from build123d import *

# Parameters (mm, degrees)
F0_W        = 105
F0_H        = 60
F1_DEPTH    = 20
F2_R        = 2.5
F3_R        = 2.5
F4_R        = 2.5
F5_T1_DEPTH = 23.75
F5_S5_W     = 2.5
F5_S5_H     = 2.5
F5_T6_DEPTH = 2.5
F6_R        = 2.5


# Not quite as in the source:
# - a fillet or chamfer that OpenCascade refuses, or shapes differently, is made with other operations: its cross-section is extruded or revolved along the edge and cut away or added


with BuildPart() as f1:
    # F0 (on Top) → F1 (new body)
    with BuildSketch(Plane.XY):
        Rectangle(F0_W, F0_H)
        with BuildLine():
            ThreePointArc((-17.4192723763, 1.0974504119), (-17.4394815095, 0.547242643), (-17.5, 0))
            ThreePointArc((-17.5, 0), (-32.3990632431, 1.6476581808), (-17.4192723763, 1.0974504119))
        make_face(mode=Mode.SUBTRACT)
        with BuildLine():
            ThreePointArc((-7.5, 0), (0, 7.5), (7.5, 0))
            ThreePointArc((7.5, 0), (0, -7.5), (-7.5, 0))
        make_face(mode=Mode.SUBTRACT)
        with BuildLine():
            ThreePointArc((32.4798090562, 0.5499604379), (25.2549745325, -6.9449901264), (17.5, 0))
            ThreePointArc((17.5, 0), (24.7046435799, 8.0449110021), (32.4798090562, 0.5499604379))
        make_face(mode=Mode.SUBTRACT)
    extrude(amount=F1_DEPTH)

    # F2
    f2_edges = [f1.edges().sort_by_distance(p)[0] for p in [
        (0, -30, 20),
    ]]
    fillet(f2_edges, radius=F2_R)

    # F3
    f3_edges = [f1.edges().sort_by_distance(p)[0] for p in [
        (52.5, 1.25, 20),
        (0, 30, 20),
    ]]
    fillet(f3_edges, radius=F3_R)

    # F4
    f4_edges = [f1.edges().sort_by_distance(p)[0] for p in [
        (-52.5, 0, 20),
    ]]
    fillet(f4_edges, radius=F4_R)

    # F5: fillet of radius 2.5 on 1 edges, made by hand

    # F5_s2 → F5_t1 (cut)
    with BuildSketch(Plane.XY.offset(-6.25)):
        with BuildLine():
            ThreePointArc((50, 30), (51.767766953, 29.267766953), (52.5, 27.5))
            Line((52.5, 27.5), (52.5, 30))
            Line((52.5, 30), (50, 30))
        make_face()
    extrude(amount=F5_T1_DEPTH, mode=Mode.SUBTRACT)


with BuildPart() as f5_tool4:
    # F5_s5 → F5_t6 (new body)
    with BuildSketch(Plane.XZ.offset(-27.5)):
        with Locations((51.25, 18.75)):
            Rectangle(F5_S5_W, F5_S5_H)
    extrude(amount=-F5_T6_DEPTH)

    # F5_s7 → F5_t8 (revolve, cut)
    with BuildSketch(Plane(origin=(50, 27.5, 17.5), x_dir=(-0.7071067812, 0, -0.7071067812), z_dir=(0.7071067812, 0, -0.7071067812))):
        with BuildLine():
            ThreePointArc((0, -2.5), (2.5, 0), (0, 2.5))
            Line((0, 2.5), (0, -2.5))
        make_face()
    revolve(axis=Axis((50, 27.5, 17.5), (0, 1, 0)), mode=Mode.SUBTRACT)


with BuildPart() as f1_1:
    add(f1.part)

    # F5_t3: cut F5_tool4
    add(f5_tool4.part, mode=Mode.SUBTRACT)

    # F6
    f6_edges = [f1_1.edges().sort_by_distance(p)[0] for p in [
        (52.5, 0, 0),
    ]]
    fillet(f6_edges, radius=F6_R)


solid = f1_1.part
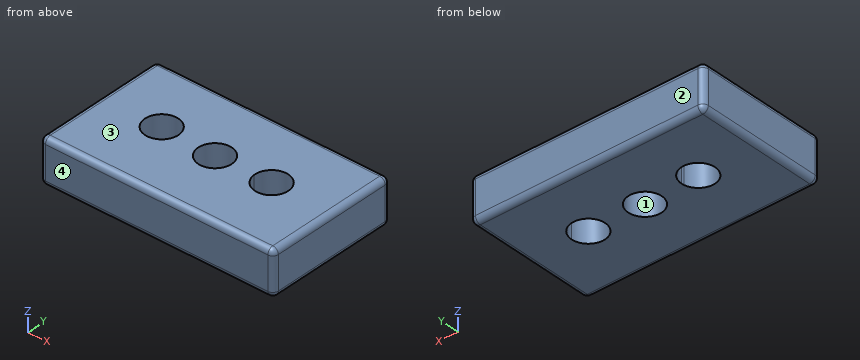
Build history of the part. All positions in model axes, mm. Face numbers are marked on the shaded views. Round coordinates to 2 decimals unless told otherwise and drop trailing zeros. Loops run counter-clockwise (first coordinate to the right, second up) from the corner with the lowest first, then second, coordinate; pieces in that order, holes last. Notation, with made-up numbers: (9, 76.25) -> (30, 76.25) arc R10 ccw to (30, 94.25) -> close; hole circle Ø4 at (18.5, 12). An arc over 180 degrees is marked (long way). Use CSV: the item, a comma, the result in double quotes. Start each with the question number.
Q1. Saw through at A-A on x = 0. Give the cut face in (y, z), and give its area (3 significant figures).
Q2. Drill centre lines: L1, parallel to Y at x = 0, z = 10.25; L2, parallel to X at y = -1, z = 19; L3, parallel to Y at x = -30.5, z = 15. Where is each one in solid material? Low to high.
Q3. Saw through at D-D on x = 22.5. Give the cut face in (y, z).
Q4. Mould opens along Y. For the marked faces 1, 2, 3 and 4 say: +Y half, -Y half, draft (parallel to the pull), parting line (faces both ways), or undercut.
Q5. Saw through at C-C on z = 13.25. Give the cut face in (x, y), and give its area (3 significant figures).
Q6. Flat gauge pin, fed straight in: pin 1 Ø13.5 at (x, y) = (-24.92, 1.1) entering from -Z. Where does the tip first touch, or does it go through?
Q7. Saw through at B-B on y = 3.5. Give the cut face in (x, z).
Solutions:
1,outline,"(-30, 2.5) arc R2.5 ccw to (-27.5, 0) -> (-7.5, 0) -> (-7.5, 20) -> (-27.5, 20) arc R2.5 ccw to (-30, 17.5) -> close; (7.5, 0) -> (27.5, 0) arc R2.5 ccw to (30, 2.5) -> (30, 17.5) arc R2.5 ccw to (27.5, 20) -> (7.5, 20) -> close"
1,area,"895 mm^2"
2,L1,"y = -30 to -7.5, 7.5 to 30"
2,L2,"x = -52 to -32.12, -17.72 to -7.43, 7.43 to 17.64, 32.32 to 52"
2,L3,"y = -30 to -3.91, 6.11 to 30"
3,outline,"(-30, 2.5) arc R2.5 ccw to (-27.5, 0) -> (-6.53, 0) -> (-6.53, 20) -> (-27.5, 20) arc R2.5 ccw to (-30, 17.5) -> close; (7.63, 0) -> (27.5, 0) arc R2.5 ccw to (30, 2.5) -> (30, 17.5) arc R2.5 ccw to (27.5, 20) -> (7.63, 20) -> close"
4,face 1,"undercut"
4,face 2,"+Y half"
4,face 3,"draft"
4,face 4,"-Y half"
5,outline,"(-52.5, -27.5) arc R2.5 ccw to (-50, -30) -> (50, -30) arc R2.5 ccw to (52.5, -27.5) -> (52.5, 27.5) arc R2.5 ccw to (50, 30) -> (-50, 30) arc R2.5 ccw to (-52.5, 27.5) -> close; hole circle Ø15 at (-24.92, 1.1); hole circle Ø15 at (0, 0); hole circle Ø15 at (24.98, 0.55)"
5,area,"5,760 mm^2"
6,pin 1,"passes through"
7,outline,"(-52.5, 2.5) arc R2.5 ccw to (-50, 0) -> (-32.02, 0) -> (-32.02, 20) -> (-50, 20) arc R2.5 ccw to (-52.5, 17.5) -> close; (-17.81, 0) -> (-6.63, 0) -> (-6.63, 20) -> (-17.81, 20) -> close; (6.63, 0) -> (18.08, 0) -> (18.08, 20) -> (6.63, 20) -> close; (31.88, 0) -> (50, 0) arc R2.5 ccw to (52.5, 2.5) -> (52.5, 17.5) arc R2.5 ccw to (50, 20) -> (31.88, 20) -> close"
